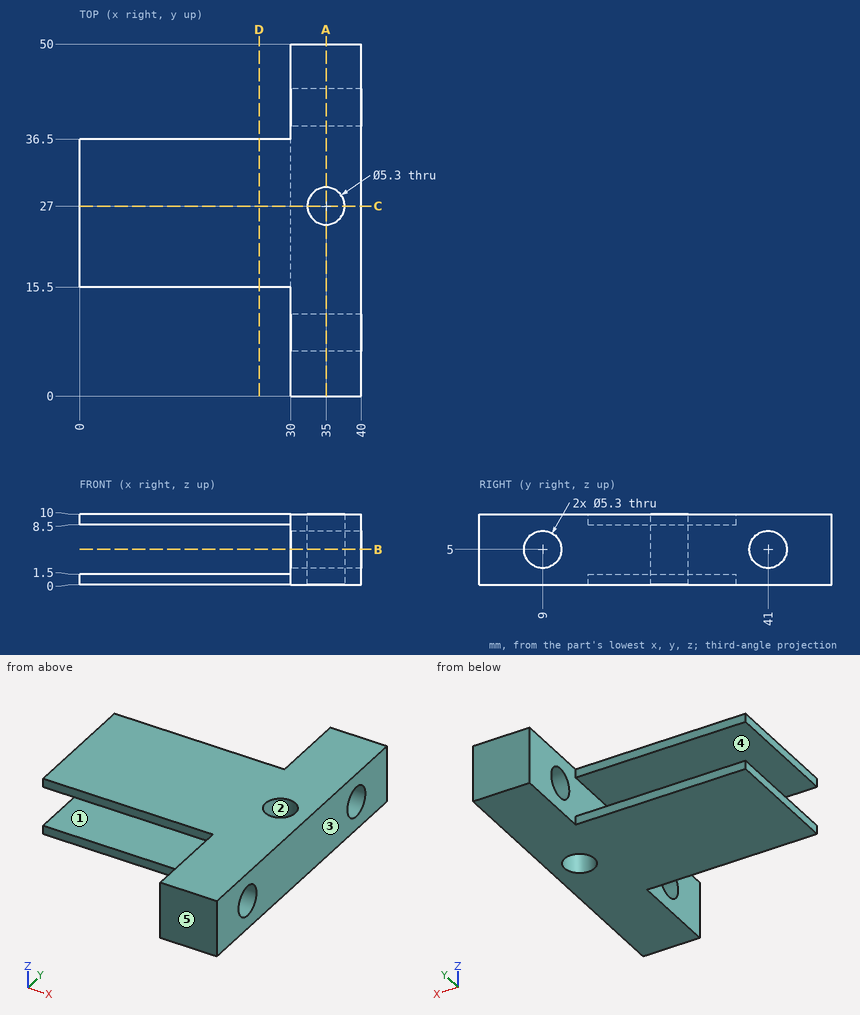
Print and shaded views of the part. All mm, measured from the part's lowest x, y and z. A direction names the side the tool comes from. Give positions to 0.01 mm unless a question says otherwise; leave off trailing zeros. Loops run counter-clockwise (first coordinate to the right, second up) from the corner with the lowest first, then second, coordinate; pieces in that order, holes last.
1) Saw through at C-C (y = 27). Write the cut outline in (x, z).
2) Saw through at A-A (x = 35). Write the cut outline in (y, z).
3) Flat gauge pins, fed straight in: pin 1 Ø1.2 at (x, z) = (12.5, 0.5) entering from -Y; pin 2 Ø1.2 at (x, z) = (21, 9.5) entering from +Y; pin 3 Ø1 at (y, z) = (45, 3.5) entering from -X; pin 4 Ø1 at (y, z) = (40.5, 3) entering from -X. Where does each tip first touch, or does it go through?
4) Pull direction X, two halves, no side cores. Call the marked faces 1, 2 and 3: +X half, -X half, draft (parallel to the pull), parting line (faces both ways), or undercut.
5) Saw through at B-B (z = 5). Write the cut outline in (x, y).
6) Tool access for the marked faces 4 and 5: list every direction of +Z, -Z, +X, -X, +Y, -Y with a clear straight run to the whole face (end or side of a thin tool).
7) Wall check: line 1 (Y direction, x = 35, z = 4.75); line 2 (Z direction, x = 16, y = 30); line 3 (Y direction, x = 35, z = 6.25). Give the ranges that are in metal, low to high.
8) Saw through at D-D (x = 25.5). Write the cut outline in (y, z), plus the area to 3 significant figures.
Answer block:
1. outline: (0, 0) - (32.35, 0) - (32.35, 10) - (0, 10) - (0, 8.5) - (30, 8.5) - (30, 1.5) - (0, 1.5) - close; (37.65, 0) - (40, 0) - (40, 10) - (37.65, 10) - close
2. outline: (0, 0) - (24.35, 0) - (24.35, 10) - (0, 10) - close; (29.65, 0) - (50, 0) - (50, 10) - (29.65, 10) - close; hole circle Ø5.3 at (9, 5); hole circle Ø5.3 at (41, 5)
3. pin 1: stops at y = 15.5
3. pin 2: stops at y = 36.5
3. pin 3: stops at x = 30
3. pin 4: passes through
4. face 1: draft
4. face 2: undercut
4. face 3: +X half
5. outline: (30, 0) - (40, 0) - (40, 6.35) - (30, 6.35) - close; (30, 11.65) - (40, 11.65) - (40, 38.35) - (30, 38.35) - close; (30, 43.65) - (40, 43.65) - (40, 50) - (30, 50) - close; hole circle Ø5.3 at (35, 27)
6. face 4: -X, +Y, -Y
6. face 5: +Z, -Z, +X, -X, -Y
7. line 1: y = 0 to 6.36, 11.64 to 24.35, 29.65 to 38.36, 43.64 to 50
7. line 2: z = 0 to 1.5, 8.5 to 10
7. line 3: y = 0 to 6.66, 11.34 to 24.35, 29.65 to 38.66, 43.34 to 50
8. outline: (15.5, 0) - (36.5, 0) - (36.5, 1.5) - (15.5, 1.5) - close; (15.5, 8.5) - (36.5, 8.5) - (36.5, 10) - (15.5, 10) - close
8. area: 63.0 mm2
